Verification items for the finished model (mm, model axes). Coordinates: 2 decimals unless noted, no trailing zeros. Order: outer loops, then holes, each group sorted by start corner. A loop starts at its lowest first (then second) coordinate and runs counter-clockwise, first axis right, second up. Notation, with made-up numbers: (1, 42) - (5, 42) arc R9 ccw to (5, 51) - close; hole circle Ø2 at (-1, 12.25). An arc over 180 degrees is marked (long way). One line per question, with ' | ' between items. Start each with the question number.
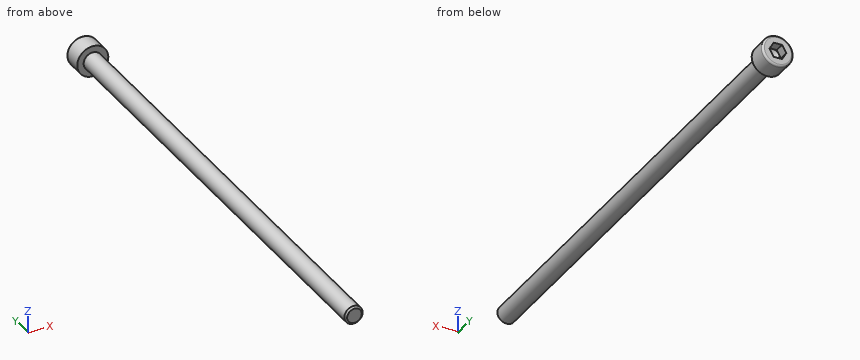
from build123d import *

# Parameters (mm, degrees)
ESQUISSE2_R             = 2.5
BASE_EXTRUSION_DEPTH    = 135
CHANFREIN1_SIZE         = 0.5
ENL_V_MAT_EXTRU_1_DEPTH = 2.75


with BuildPart() as part:
    # Esquisse2 → Base-Extrusion (new body)
    with BuildSketch(Plane(origin=(0, 0, 0), x_dir=(1, 0, 0), z_dir=(0, 1, 0))):
        with Locations(Location((0, 0, 0), (0, 0, 270))):  # turned: the seam where the file's is
            Circle(ESQUISSE2_R)
    extrude(amount=-BASE_EXTRUSION_DEPTH)

    # Chanfrein1
    chanfrein1_edges = [part.edges().sort_by_distance(p)[0] for p in [
        (0, -135, -2.5),
    ]]
    chamfer(chanfrein1_edges, length=CHANFREIN1_SIZE)

    # Esquisse5 → Boss.-Révol.1 (revolve)
    with BuildSketch(Plane.XY, mode=Mode.PRIVATE) as boss_r_vol_1_sk:
        with BuildLine():
            Line((2, 5.5), (2, 2.75))
            Line((2, 2.75), (0, 1.595299462))
            Line((0, 1.595299462), (0, 0))
            Line((0, 0), (4.25, 0))
            Line((4.25, 0), (4.25, 4.95))
            ThreePointArc((4.25, 4.95), (4.08890873, 5.33890873), (3.7, 5.5))
            Line((3.7, 5.5), (2, 5.5))
        make_face()
    revolve(boss_r_vol_1_sk.sketch.rotate(Axis((0, 5.5, 0), (0, -1, 0)), 90), axis=Axis((0, 5.5, 0), (0, -1, 0)))  # turned: the seam where the file's is

    # Esquisse7 → Enlèv. mat.-Extru.1 (cut)
    with BuildSketch(Plane(origin=(0, 5.5, 0), x_dir=(-1, 0, 0), z_dir=(0, 1, 0))):
        Polygon((1.154700538, 2), (-1.154700538, 2), (-2.309401077, 0), (-1.154700538, -2), (1.154700538, -2), (2.309401077, 0), align=None)
    extrude(amount=-ENL_V_MAT_EXTRU_1_DEPTH, mode=Mode.SUBTRACT)


solid = part.part
Item 1: Gauge pin test, flat ends, axial feed: pin 1 (3 mm diameter, centred on y = -39, z = -0.5, fed in from -X); pin 2 (2 mm diameter, centred on x = -1, y = -84.5, fed in from -Z); pin 3 (1.5 mm diameter, centred on y = -83.5, z = 3, fed in from +X). Record the tip position at first contact, or that the pin passes through.
Item 2: Thickness scan on probe 1 along Z at (x, y) = (0.25, -74); probe 2 along X at (y, z) = (-28, 1); probe 3 along Y at (x, z) = (-2.5, -2.75). Record the ranges inside material, lowest first. Write a range as from..to.
Item 3: Section check A-A (y = -15). Record the cut outline in (x, z), then the cut area to 3 significant figures.
Completed:
1) pin 1: stops at x = -2.5 | pin 2: stops at z = -2.5 | pin 3: stops at x = 1.09
2) probe 1: z = -2.49..2.49 | probe 2: x = -2.29..2.29 | probe 3: y = 0..5.5
3) outline: circle Ø5 at (0, 0) | area: 19.6 mm^2
